```python
from build123d import *

# Parameters (mm, degrees)
SKETCH3_W           = 1219.2
SKETCH3_H           = 608.0125
BOSS_EXTRUDE1_DEPTH = 20.6375
SKETCH4_W           = 1219.2
SKETCH4_H           = 608.0125
SKETCH4_W_2         = 1146.175
SKETCH4_H_2         = 534.9875
BOSS_EXTRUDE2_DEPTH = 136.525
SKETCH5_W           = 1146.175
SKETCH5_H           = 534.9875
SKETCH5_W_2         = 1073.15
SKETCH5_H_2         = 461.9625
BOSS_EXTRUDE3_DEPTH = 98.425
SKETCH6_W           = 87.3125
SKETCH6_H           = 461.9625
BOSS_EXTRUDE4_DEPTH = 60.325
SKETCH7_W           = 50.8
SKETCH7_H           = 38.1
CUT_EXTRUDE1_DEPTH  = 549.275
SKETCH8_R           = 15.875
CUT_EXTRUDE2_DEPTH  = 73.025


with BuildPart() as part:
    # Sketch3 → Boss-Extrude1 (new body)
    with BuildSketch(Plane(origin=(0, 0, 0), x_dir=(1, 0, 0), z_dir=(0, 1, 0))):
        with Locations((609.6, 304.00625)):
            Rectangle(SKETCH3_W, SKETCH3_H)
    extrude(amount=BOSS_EXTRUDE1_DEPTH)

    # Sketch4 → Boss-Extrude2 (add)
    with BuildSketch(Plane(origin=(0, 20.6375, 0), x_dir=(1, 0, 0), z_dir=(0, 1, 0))):
        with Locations((609.6, 304.00625)):
            Rectangle(SKETCH4_W, SKETCH4_H)
        with Locations((609.6, 304.00625)):
            Rectangle(SKETCH4_W_2, SKETCH4_H_2, mode=Mode.SUBTRACT)
    extrude(amount=BOSS_EXTRUDE2_DEPTH)

    # Sketch5 → Boss-Extrude3 (add)
    with BuildSketch(Plane(origin=(0, 20.6375, 0), x_dir=(1, 0, 0), z_dir=(0, 1, 0))):
        with Locations((609.6, 304.00625)):
            Rectangle(SKETCH5_W, SKETCH5_H)
        with Locations((609.6, 304.00625)):
            Rectangle(SKETCH5_W_2, SKETCH5_H_2, mode=Mode.SUBTRACT)
    extrude(amount=BOSS_EXTRUDE3_DEPTH)

    # Sketch6 → Boss-Extrude4 (add)
    with BuildSketch(Plane(origin=(0, 20.6375, 0), x_dir=(1, 0, 0), z_dir=(0, 1, 0))):
        with Locations((843.75625, 304.00625)):
            Rectangle(SKETCH6_W, SKETCH6_H)
        with Locations((381.79375, 304.00625)):
            Rectangle(SKETCH6_W, SKETCH6_H)
    extrude(amount=BOSS_EXTRUDE4_DEPTH)

    # Sketch7 → Cut-Extrude1 (cut)
    with BuildSketch(Plane(origin=(887.4125, 0, 0), x_dir=(0, 0, -1), z_dir=(1, 0, 0))):
        with Locations((301.625, 39.6875)):
            Rectangle(SKETCH7_W, SKETCH7_H)
    extrude(amount=-CUT_EXTRUDE1_DEPTH, mode=Mode.SUBTRACT)

    # Sketch8 → Cut-Extrude2 (cut)
    with BuildSketch(Plane(origin=(73.025, 0, 0), x_dir=(0, 0, -1), z_dir=(1, 0, 0))):
        with Locations((468.3125, 74.6125)):
            Circle(SKETCH8_R)
    extrude(amount=-CUT_EXTRUDE2_DEPTH, mode=Mode.SUBTRACT)


solid = part.part
```
Geometry check sheet. Reference: the model listing, model coordinates, mm. A direction names the side the tool comes from. Give positions to 0.01 mm unless a question says otherwise; leave off trailing zeros. Loops run counter-clockwise (first coordinate to the right, second up) from the corner with the lowest first, then second, coordinate; pieces in that order, holes last. Notation, with made-up numbers: (73.25, 7) - (92.25, 7) arc R12 ccw to (92.25, 16) - close; hole circle Ø9 at (6, 79.5). An arc over 180 degrees is marked (long way). Use CSV: the item, a comma, the result in double quotes. Start each with the question number.
Q1. Section check D-D, the plane x = 384. Record the cut outline in (y, z) (1 decimal).
Q2. Section check C-C, the plane x = 779. Record the cut outline in (y, z) (1 decimal).
Q3. Release check for a two-part mould opening along X. For faces 4 (the face through (601, 77, -608.012)), 5 (the face through (0, 77, -300)), 6 (the face through (1219.2, 77, -300)), 7 (the face through (602, 138, -571.5)) record: +X half, -X half, draft (parallel to the pull), parting line (faces both ways), or undercut.
Q4. Section check A-A, the plane z = -293.5. Count the separate pieces of the cut face and the enclosed holes in it, and give its area (3 significant figures).
Q5. Access from +Z, -Z, +X, -X, +Y, -Y to the whole of each face (thin tool, end or side, straight path). Record for faces 1 (the face through (382, 58.738, -301)), 2 (the face through (37.024, 87.998, -476.847)), 3 (the face through (1146.175, 69, -301)).
Q6. Go/stop test with a flat-tipped pin: pin 1 Ø3 at (x, z) = (282, -115) entering from +Y. Record where the tip stops, or that it passes through.
Q7. Scan lines: probe 1 along X at (y, z) = (134, -385.5); probe 2 along X at (y, z) = (117, -530.5) (3 decimals); probe 3 along Z at (x, y) = (232.5, 131). Record each from-to range of solid material in increasing order. Write a range as from..to.
Findings below:
1,outline,"(0, -608) - (157.2, -608) - (157.2, -571.5) - (119.1, -571.5) - (119.1, -535) - (81, -535) - (81, -73) - (119.1, -73) - (119.1, -36.5) - (157.2, -36.5) - (157.2, 0) - (0, 0) - close; hole (20.6, -327) - (58.7, -327) - (58.7, -276.2) - (20.6, -276.2) - close"
2,outline,"(0, -608) - (157.2, -608) - (157.2, -571.5) - (119.1, -571.5) - (119.1, -535) - (20.6, -535) - (20.6, -73) - (119.1, -73) - (119.1, -36.5) - (157.2, -36.5) - (157.2, 0) - (0, 0) - close"
3,face 4,"draft"
3,face 5,"-X half"
3,face 6,"+X half"
3,face 7,"undercut"
4,separate pieces,"3"
4,enclosed holes,"0"
4,area,"46,200 mm^2"
5,face 1,"none"
5,face 2,"-X"
5,face 3,"+Y"
6,pin 1,"stops at y = 20.64"
7,probe 1,"x = 0..36.51, 1182.69..1219.2"
7,probe 2,"x = 0..73.025, 1146.175..1219.2"
7,probe 3,"z = -608.01..-571.5, -36.51..0"
